Design review of the part built by this model. Coordinates are the model's own, in mm. Round coordinates to 2 decimals unless told otherwise and drop trailing zeros. Write each loop counter-clockwise with the first axis right and the second up, starting at its lowest first coordinate (ties: lowest second). Pieces come first, ordered by that corner, then holes. Notation, with made-up numbers: (66.5, -14.75) -> (77.5, -14.75) arc R19 ccw to (77.5, 1.25) -> close; hole circle Ø3 at (88, 85). An arc over 180 degrees is marked (long way). Write item = value, one per line. Start each with the question number.
Item 1: Add section B-B, the plane x = 47.5. State the section outline as (y, z) points, then the cut area to 3 significant figures.
Item 2: To check wall thickness, follow L1, parallel to Z at x = 92, y = -130; L2, parallel to Y at x = 38, z = -28; L3, parallel to Z at x = 22, y = -431. State the ranges of each line that lie inside material, in increasing order.
Item 3: For pin 1 Ø25 at (x, z) = (59.5, 10) entering from -Y; pin 2 Ø1 at (x, y) = (43, 149) entering from -Z; pin 3 Ø14 at (x, y) = (72.5, 6.5) entering from -Z, all flat-tipped, find the tip position at first contact; note any pin that passes through.
Item 4: Add section A-A, the plane z = 0. State the section outline as (x, y) points, then the cut area to 3 significant figures.
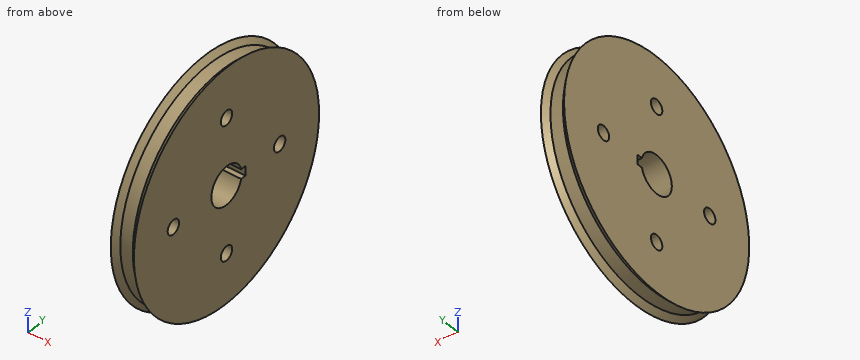
Autodesk Inventor part; units mm, degrees
ref_plane "YZ Plane" through (0, 0, 0) normal (1, 0, 0) x (0, 1, 0)
ref_plane "XZ Plane" through (0, 0, 0) normal (0, 1, 0) x (-1, 0, 0)
ref_plane "XY Plane" through (0, 0, 0) normal (0, 0, 1) x (1, 0, 0)
sketch "Sketch1" plane through (0, 0, 0) normal (0, 0, 1) x (1, 0, 0)
  line L0 (0, 0) -> (100, 0)
  line L1 (100, 0) -> (100, 500)
  line L2 (0, 500) -> (0, 0)
  line L3 (0, 500) -> (17.6777, 482.3223)
  line L4 (0, 500) -> (25, 500) construction
  line L5 (100, 500) -> (82.3223, 482.3223)
  line L6 (100, 500) -> (125, 500) construction
  line L7 (82.3223, 482.3223) -> (17.6777, 482.3223)
  line L8 (50, -100) -> (-150, -100)
  dimension "d7" = 200
revolve "Revolution1" add sketch "Sketch1" angle 360 about axis through (50, -100, 0) along (-1, 0, 0)
sketch "Sketch2" plane through (0, -100, 0) normal (-1, 0, 0) x (0, 0, 1)
  circle A0 centre (0, 0) radius 600
  circle A1 centre (350, 0) radius 37.5
  circle A2 centre (0, 0) radius 100
  circle A3 centre (0, -350) radius 37.5
  circle A4 centre (-350, 0) radius 37.5
  circle A5 centre (0, 350) radius 37.5
  point P0 (0, 100)
  dimension "d9" = 75
  dimension "d12" = 360
extrude "Extrusion1" cut sketch "Sketch2" against normal blind 200 contours A1 | A3 | A4 | A5
thicken "Thicken1" operation add thickness 10 both sides no extend neighbours yes toward (1, 0, 0) faces at (100, -364.9419, 262.9039)
thicken "Thicken2" operation add thickness 10 both sides no extend neighbours yes toward (-1, 0, 0) faces at (0, -364.9419, 262.9039)
sketch "Sketch3" plane through (-10, -100, 0) normal (-1, 0, 0) x (0, 0, 1)
  line L0 (25, 96.8246) -> (25, 125)
  line L1 (25, 125) -> (-25, 125)
  line L2 (-25, 125) -> (-25, 96.8246)
  line L3 (-25, 75) -> (25, 125) construction
  line L4 (25, 75) -> (-25, 125) construction
  circle A0 centre (0, 0) radius 100
  circle A1 centre (0, 0) radius 100
  point P0 (0, 100)
extrude "Extrusion2" cut sketch "Sketch3" against normal blind 120 contours A0 L2 L1 L0
properties part number "Practica 2 Polea"
Result set:
q1.outline = circle Ø1164.64 at (-100, 0); hole circle Ø75 at (-450, 0); hole circle Ø75 at (-100, -350); hole circle Ø75 at (-100, 350); hole (-3.18, -25) -> (25, -25) -> (25, 25) -> (-3.18, 25) arc R100 ccw (long way) to start; hole circle Ø75 at (250, 0)
q1.area = 1,010,000 mm²
q2.L1 = -591.24 to -372.5, -327.5 to -95.39, 95.39 to 327.5, 372.5 to 591.24
q2.L2 = -681.65 to -474.94, -425.06 to -196, -4 to 225.06, 274.94 to 481.65
q2.L3 = -479.1 to -32.33, 32.33 to 479.1
q3.pin_1 = -682.32
q3.pin_2 = -526.64
q3.pin_3 = -573.76
q4.outline = (-10, -710) -> (17.68, -682.32) -> (82.32, -682.32) -> (110, -710) -> (110, -487.5) -> (-10, -487.5) -> close; (-10, -412.5) -> (110, -412.5) -> (110, -200) -> (-10, -200) -> close; (-10, 25) -> (110, 25) -> (110, 212.5) -> (-10, 212.5) -> close; (-10, 287.5) -> (110, 287.5) -> (110, 510) -> (82.32, 482.32) -> (17.68, 482.32) -> (-10, 510) -> close
q4.area = 96,300 mm²
